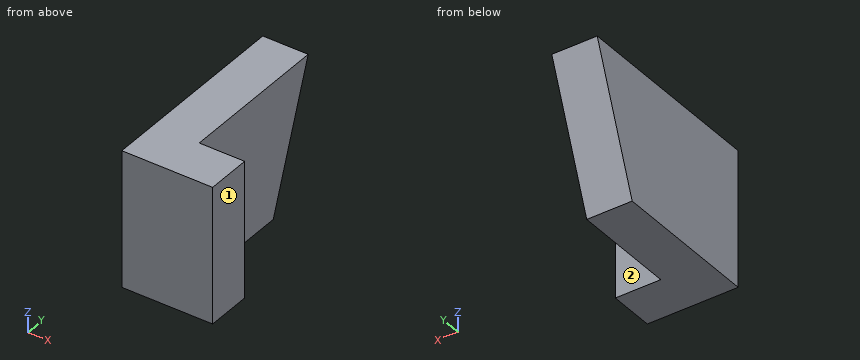
from build123d import *

# Parameters (mm, degrees)
BOSS_EXTRUDE1_DEPTH = 15
CUT_EXTRUDE1_DEPTH  = 10


with BuildPart() as part:
    # Sketch1 → Boss-Extrude1 (new body)
    with BuildSketch(Plane.XY):
        Polygon((0, 0), (0, 25), (5, 25), (5, 5), (10, 5), (10, 0), align=None)
    extrude(amount=BOSS_EXTRUDE1_DEPTH)

    # Sketch2 → Cut-Extrude1 (cut)
    with BuildSketch(Plane(origin=(5, 0, 0), x_dir=(0, 0, -1), z_dir=(1, 0, 0))):
        Polygon((-15, 22.026317018), (-18.328083999, 30.478992543), (8.324959991, 29.895957206), (0, 16.566763504), align=None)
    extrude(amount=-CUT_EXTRUDE1_DEPTH, mode=Mode.SUBTRACT)


solid = part.part
Geometry check sheet. Reference: the model listing, model coordinates, mm. Face numbers are marked on the shaded views. A direction names the side the tool comes from. Give positions to 0.01 mm unless a question says otherwise; leave off trailing zeros. Write each loop counter-clockwise with the first axis right and the second up, starting at its lowest first coordinate (ties: lowest second). Pieces come first, ordered by that corner, then holes.
1) Cross-section at C-C (y = 15.25). Record the boundary of the cut face in (x, z), plus the area to 3 significant figures.
Values follow:
outline: (0, 0) - (5, 0) - (5, 15) - (0, 15) - close
area: 75.0 mm2
2) Go/stop test with flat-tipped pins: pin 1 Ø1 at (x, y) = (6.5, 16.5) entering from -Z; pin 2 Ø6 at (x, z) = (1.5, 5.5) entering from +Y; pin 3 Ø2.5 at (x, z) = (8.5, 11) entering from +Y. Record where each tip stops, or that it passes through.
Values follow:
pin 1: passes through
pin 2: stops at y = 19.66
pin 3: stops at y = 5
3) Set-up check for the marked faces 1 and 2: record each of +Z, -Z, +X, -X, +Y, -Y from which the full face is reachable in a straight line by a thin tool's end or side.
Values follow:
face 1: +Z, -Z, +X, +Y, -Y
face 2: +Z, -Z, +X, +Y
4) Cross-section at D-D (z = 10.75). Record the boundary of the cut face in (x, y).
Values follow:
outline: (0, 0) - (10, 0) - (10, 5) - (5, 5) - (5, 20.48) - (0, 20.48) - close
5) Cross-section at A-A (x = 4.75). Record the boundary of the cut face in (y, z), plus the area to 3 significant figures.
Values follow:
outline: (0, 0) - (16.57, 0) - (22.03, 15) - (0, 15) - close
area: 289 mm2
6) Thickness scan on line 1 (X direction, y = 18, z = 4.5); line 2 (Y direction, x = 2.75, z = 3). Record the ranges inside material, lowest first.
Values follow:
line 1: x = 0 to 5
line 2: y = 0 to 17.66
7) Cross-section at B-B (z = 8.75). Record the boundary of the cut face in (x, y).
Values follow:
outline: (0, 0) - (10, 0) - (10, 5) - (5, 5) - (5, 19.75) - (0, 19.75) - close
